For this review, take the finished solid that the model builds, in its own axes (mm). A direction names the side the tool comes from. Give positions to 0.01 mm unless a question says otherwise; leave off trailing zeros. Write each loop counter-clockwise with the first axis right and the second up, starting at its lowest first coordinate (ties: lowest second). Pieces come first, ordered by that corner, then holes.
from build123d import *

# Parameters (mm, degrees)
F1_DEPTH    = 99.5
F2_T        = -1.1
F3_R        = 3
F4_W        = 6
F4_H        = 3
F5_DEPTH    = 1
F6_T4_DEPTH = 31.981320863
F7_W        = 6
F7_H        = 3
F8_DEPTH    = 1
F9_T4_DEPTH = 31.981320863


# Not quite as in the source:
# - a fillet or chamfer that OpenCascade refuses, or shapes differently, is made with other operations: its cross-section is extruded or revolved along the edge and cut away or added


with BuildPart() as f1:
    # F0 (on Right) → F1 (new body)
    with BuildSketch(Plane.YZ):
        Polygon((-49.5, 0), (0, 0), (0, 12), (-45, 62), (-45, 122), (-75, 157), (-75, 122), (-74, 121), (-74, 56), (-49.5, 5), align=None)
    extrude(amount=F1_DEPTH)

    # F2
    f2_openings = [f1.faces().sort_by_distance(p)[0] for p in [
        (49.75, -75, 139.5),
        (49.75, -24.75, 0),
    ]]
    offset(amount=F2_T, openings=f2_openings, kind=Kind.INTERSECTION)

    # F3
    f3_edges = [f1.edges().sort_by_distance(p)[0] for p in [
        (49.75, -74, 121),
        (49.75, -74, 56),
        (49.75, -49.5, 5),
        (49.75, 0, 12),
        (49.75, -45, 62),
        (49.75, -45, 122),
        (49.75, -1.1, 11.57789),
        (49.75, -46.1, 61.57789),
        (49.75, -72.9, 56.250512),
        (49.75, -46.1, 121.593084),
        (49.75, -72.9, 121.455635),
        (49.75, -48.4, 5.250512),
    ]]
    fillet(f3_edges, radius=F3_R)

    # F4 (on face) → F5 (join)
    with BuildSketch(Plane(origin=(0, 0, 0), x_dir=(0, -1, 0), z_dir=(-1, 0, 0))):
        with Locations((25, 4.5)):
            Rectangle(F4_W, F4_H)
    extrude(amount=F5_DEPTH)

    # F6: chamfer of 1 x 5 on 1 edges, made by hand


with BuildPart() as f6_tool2:
    # F6_s3 → F6_t4 (new body)
    with BuildSketch(Plane.XZ.offset(40.9906604315)):
        Polygon((0, 6), (-1, 1), (-1, 6), align=None)
    extrude(amount=-F6_T4_DEPTH)

    split(bisect_by=Plane.YZ, keep=Keep.BOTTOM)


with BuildPart() as f1_1:
    add(f1.part)

    # F6_t1: cut F6_tool2
    add(f6_tool2.part, mode=Mode.SUBTRACT)

    # F7 (on face) → F8 (join)
    with BuildSketch(Plane.YZ.offset(99.5)):
        with Locations((-25, 4.5)):
            Rectangle(F7_W, F7_H)
    extrude(amount=F8_DEPTH)

    # F9: chamfer of 1 x 5 on 1 edges, made by hand


with BuildPart() as f9_tool2:
    # F9_s3 → F9_t4 (new body)
    with BuildSketch(Plane.XZ.offset(9.0093395685)):
        Polygon((99.5, 6), (100.5, 1), (100.5, 6), align=None)
    extrude(amount=F9_T4_DEPTH)

    split(bisect_by=Plane.YZ.offset(99.5), keep=Keep.TOP)


with BuildPart() as f1_2:
    add(f1_1.part)

    # F9_t1: cut F9_tool2
    add(f9_tool2.part, mode=Mode.SUBTRACT)


solid = f1_2.part
(1) Clearance check with flat-ended pins moving along their axes: pin 1 Ø17.5 at (x, z) = (64.5, 85.5) entering from -Y; pin 2 Ø4 at (x, z) = (75, 135) entering from -Y; pin 3 Ø12 at (y, z) = (-57, 89) entering from +X; pin 4 Ø1.4 at (x, z) = (36.5, 3) entering from +Y. State where each tip first meets the part, or that it passes through.
(2) For L1, parallel to X at y = -53, z = 119; L2, parallel to Y at x = 44.5, z = 73; L3, parallel to Z at x = 8, y = -58, list the stretches that pass through material, from the lowest coordinate up.
(3) We need section D-D (y = -25.5). Write out the cut boundary in (x, z), and give its area (3 significant figures).
(4) We need section B-B (z = 79). Write out the cut boundary in (x, y).
(5) We need section C-C (y = -60). Write out the cut boundary in (x, z), and give its area (3 significant figures).
(6) The part is to be moulded in two halves that separate along X. For faces 6 (the flat face through (50, -75, 156)), 7 (the flat face through (49, -46.1, 91)), say which applies: +X half, -X half, draft (parallel to the pull), parting line (faces both ways), or undercut.
(7) Tool access review of faces 1 (the flat face through (50, -49, 0)), 2 (the flat face through (49.069, -23.296, 36.24)), 3 (the flat face through (98.4, -47, 61)), 4 (the flat face through (49.054, -22.196, 36.662)), 5 (the flat face through (49, -74, 89)): name each direction out of +Z, -Z, +X, -X, +Y, -Y from which nothing blocks a thin tool from reaching the whole face with its end or side.
The answers:
1. pin 1: stops at y = -74
1. pin 2: stops at y = -59.31
1. pin 3: stops at x = 99.5
1. pin 4: stops at y = 0
2. L1: x = 0 to 1.1, 98.4 to 99.5
2. L2: y = -74 to -72.9, -46.1 to -45
2. L3: z = 22.69 to 25.23, 135.48 to 137.17
3. outline: (-0.6, 3) - (0, 3) - (0, 0) - (1.1, 0) - (1.1, 38.69) - (98.4, 38.69) - (98.4, 0) - (99.5, 0) - (99.5, 3) - (100.1, 3) - (99.5, 6) - (99.5, 40.33) - (0, 40.33) - (0, 6) - close
3. area: 251 mm2
4. outline: (0, -74) - (99.5, -74) - (99.5, -45) - (0, -45) - close; hole (1.1, -72.9) - (98.4, -72.9) - (98.4, -46.1) - (1.1, -46.1) - close
5. outline: (0, 26.86) - (99.5, 26.86) - (99.5, 139.5) - (0, 139.5) - close; hole (1.1, 29.4) - (98.4, 29.4) - (98.4, 137.81) - (1.1, 137.81) - close
5. area: 659 mm2
6. face 6: draft
6. face 7: undercut
7. face 1: -Z, +X, -X, +Y, -Y
7. face 2: -Z
7. face 3: none
7. face 4: +Z, +X, -X, +Y
7. face 5: -Z, +X, -X, -Y
